from build123d import *

# Parameters (mm, degrees)
F1_DEPTH = 6.35


with BuildPart() as f1:
    # F0 (on Front) → F1 (new body)
    with BuildSketch(Plane.XZ):
        with BuildLine():
            Line((-69.944234, -6.604), (-69.944234, 0))
            Line((-69.944234, 0), (-54.704234, 0))
            Line((-54.704234, 0), (-54.704234, 21.365997))
            ThreePointArc((-54.704234, 21.365997), (-50.546907, 31.402673), (-40.510231, 35.56))
            Line((-40.510231, 35.56), (-3.175, 35.56))
            Line((-3.175, 35.56), (-3.175, 51.4096))
            Line((-3.175, 51.4096), (3.175, 51.4096))
            Line((3.175, 51.4096), (3.175, 35.56))
            Line((3.175, 35.56), (40.510231, 35.56))
            ThreePointArc((40.510231, 35.56), (50.546907, 31.402673), (54.704234, 21.365997))
            Line((54.704234, 21.365997), (54.704234, 0))
            Line((54.704234, 0), (69.944234, 0))
            Line((69.944234, 0), (69.944234, -6.604))
            Line((69.944234, -6.604), (80.104234, -6.604))
            Line((80.104234, -6.604), (80.104234, 0))
            Line((80.104234, 0), (94.074234, 0))
            Line((94.074234, 0), (94.074234, 3.265747))
            ThreePointArc((94.074234, 3.265747), (78.440691, 41.008457), (40.697981, 56.642))
            Line((40.697981, 56.642), (-40.697981, 56.642))
            ThreePointArc((-40.697981, 56.642), (-78.440691, 41.008457), (-94.074234, 3.265747))
            Line((-94.074234, 3.265747), (-94.074234, 0))
            Line((-94.074234, 0), (-80.104234, 0))
            Line((-80.104234, 0), (-80.104234, -6.604))
            Line((-80.104234, -6.604), (-69.944234, -6.604))
        make_face()
    extrude(amount=F1_DEPTH)


solid = f1.part
For this review, take the finished solid that the model builds, in its own axes (mm). A direction names the side the tool comes from. Round coordinates to 2 decimals unless told otherwise and drop trailing zeros. Order: outer loops, then holes, each group sorted by start corner. A loop starts at its lowest first (then second) coordinate and runs counter-clockwise, first axis right, second up. Notation, with made-up numbers: M 67.5,79 L 119.5,79 A24 ccw 119.5,93 Z; hole C 74,6 d10. An arc over 180 degrees is marked long. Use a Markdown table: item, result. Add a question column.
Item 1: Mouldability with a two-part tool opening along X and no side actions: class faces 1 (the cylindrical face through (78.853, -3.131, 40.591)), 2 (the flat face through (22, -3, 35.56)), 3 (the flat face through (75, -3, -6.604)), 4 (the cylindrical face through (-78.023, -3.131, 41.421)) as released by +X, released by -X, zero draft, split by the parting line, or undercut.
Item 2: Add section C-C, the plane z = 48. Give the boundary of the cut face in (x, y) (3 decimals).
Item 3: To check wall thickness, follow line 1 along X through (y, z) = (-4, 1); line 2 along Z through (x, y) = (-16, -3.75); line 3 along Z through (x, y) = (-3, -3.5). State the ranges of each line that lie inside material, in increasing order.
Item 4: Add section D-D, the plane x = 24. Give the boundary of the cut face in (y, z), then the cut area to 3 significant figures.
Item 5: Add section A-A, the plane z = 11. Give the boundary of the cut face in (x, y), then the cut area to 3 significant figures.
Item 6: Insertion check: pin 1 (4 mm diameter, centred on x = 41, z = 32, fed in from -Y); pin 2 (1.9 mm diameter, centred on x = -17.5, y = -4.5, fed in from -Z); pin 3 (3 mm diameter, centred on y = -2, z = 7, fed in from -X); pin 4 (1.9 mm diameter, centred on y = -4, z = -4.5, fed in from -X). Each pin has a flat end and moves straight along its axis. Give the tip position at first contact, or say it passes through.
Item 7: Tool access review of faces 5 (the flat face through (-80.104, -3, -3)), 6 (the flat face through (-75, -3, -6.604)), 7 (the flat face through (-54.704, -3, 11)): name each direction out of +Z, -Z, +X, -X, +Y, -Y from which nothing blocks a thin tool from reaching the whole face with its end or side.
Item 8: Add section B-B, the plane y = -4. Give the boundary of the cut face in (x, z) (1 decimal), then the cut area to 3 significant figures.
Geometry results:
| question | item | result |
|---|---|---|
| 1 | face 1 | released by +X |
| 1 | face 2 | undercut |
| 1 | face 3 | zero draft |
| 1 | face 4 | released by -X |
| 2 | outline | M -69.816,-6.35 L -3.175,-6.35 L -3.175,0 L -69.816,0 Z; M 3.175,-6.35 L 69.816,-6.35 L 69.816,0 L 3.175,0 Z |
| 3 | line 1 | x = -94.07 to -54.7, 54.7 to 94.07 |
| 3 | line 2 | z = 35.56 to 56.64 |
| 3 | line 3 | z = 51.41 to 56.64 |
| 4 | outline | M -6.35,35.56 L 0,35.56 L 0,56.64 L -6.35,56.64 Z |
| 4 | area | 134 mm² |
| 5 | outline | M -93.51,-6.35 L -54.7,-6.35 L -54.7,0 L -93.51,0 Z; M 54.7,-6.35 L 93.51,-6.35 L 93.51,0 L 54.7,0 Z |
| 5 | area | 493 mm² |
| 6 | pin 1 | passes through |
| 6 | pin 2 | stops at z = 35.56 |
| 6 | pin 3 | stops at x = -94.03 |
| 6 | pin 4 | stops at x = -80.1 |
| 7 | face 5 | -Z, -X, +Y, -Y |
| 7 | face 6 | -Z, +X, -X, +Y, -Y |
| 7 | face 7 | -Z, +Y, -Y |
| 8 | outline | M -94.1,0 L -80.1,0 L -80.1,-6.6 L -69.9,-6.6 L -69.9,0 L -54.7,0 L -54.7,21.4 A14.2 cw -40.5,35.6 L -3.2,35.6 L -3.2,51.4 L 3.2,51.4 L 3.2,35.6 L 40.5,35.6 A14.2 cw 54.7,21.4 L 54.7,0 L 69.9,0 L 69.9,-6.6 L 80.1,-6.6 L 80.1,0 L 94.1,0 L 94.1,3.3 A53.4 ccw 40.7,56.6 L -40.7,56.6 A53.4 ccw -94.1,3.3 Z |
| 8 | area | 5,660 mm² |
